The model under review builds one solid part; all positions refer to its coordinate system, in mm. Coordinates: 2 decimals unless noted, no trailing zeros. Loops run counter-clockwise (first coordinate to the right, second up) from the corner with the lowest first, then second, coordinate; pieces in that order, holes last. Notation, with made-up numbers: (-21, -21.75) - (-15, -21.75) arc R13 cw to (-15, -5.75) - close; hole circle Ø9 at (35.5, 67.5). An arc over 180 degrees is marked (long way). Use a Markdown table: item, result. Add a question column.
1) Add section A-A, the plane y = 0. Give the boundary of the cut face in (x, z) (3 decimals), and give its area (3 significant figures).
2) Add section B-B, the plane x = 225. Give the boundary of the cut face in (y, z) (3 decimals).
3) To check wall thickness, follow L1, parallel to Y at x = -225, z = 2; L2, parallel to X at y = 4, z = 3.75; L3, parallel to Y at x = 236, z = 0. State the ranges of each line that lie inside material, in increasing order. Write a range as [from, to].
4) Add section C-C, the plane z = 3. Give the boundary of the cut face in (x, y), and give its area (3 significant figures).
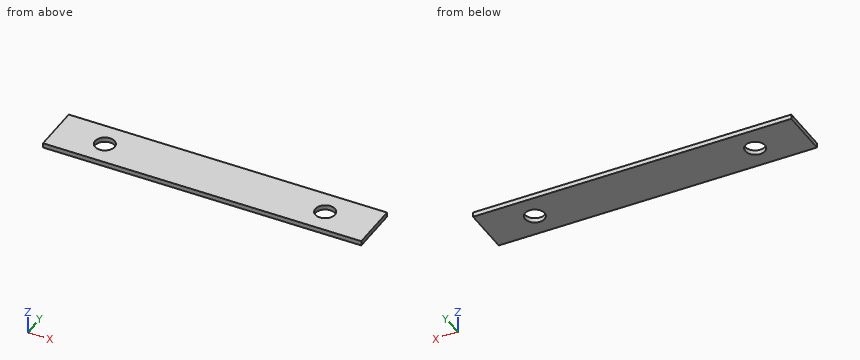
```python
from build123d import *

# Parameters (mm, degrees)
CROQUIS1_W              = 650
CROQUIS1_H              = 100
SALIENTE_EXTRUIR1_DEPTH = 4.765
CROQUIS4_R              = 20
CORTAR_EXTRUIR3_DEPTH   = 15
CROQUIS3_R              = 20
CORTAR_EXTRUIR4_DEPTH   = 15


with BuildPart() as part:
    # Croquis1 → Saliente-Extruir1 (new, symmetric)
    with BuildSketch(Plane.XY):
        Rectangle(CROQUIS1_W, CROQUIS1_H)
    extrude(amount=SALIENTE_EXTRUIR1_DEPTH, both=True)

    # Croquis4 → Cortar-Extruir3 (cut)
    with BuildSketch(Plane(origin=(0, 0, -4.765), x_dir=(-1, 0, 0), z_dir=(0, 0, -1))):
        with Locations((225, 0)):
            Circle(CROQUIS4_R)
    extrude(amount=-CORTAR_EXTRUIR3_DEPTH, mode=Mode.SUBTRACT)

    # Croquis3 → Cortar-Extruir4 (cut)
    with BuildSketch(Plane.XY.offset(4.765)):
        with Locations((225, 0)):
            Circle(CROQUIS3_R)
    extrude(amount=-CORTAR_EXTRUIR4_DEPTH, mode=Mode.SUBTRACT)


solid = part.part
```
From the geometry:
| question | item | result |
|---|---|---|
| 1 | outline | (-325, -4.765) - (-245, -4.765) - (-245, 4.765) - (-325, 4.765) - close; (-205, -4.765) - (205, -4.765) - (205, 4.765) - (-205, 4.765) - close; (245, -4.765) - (325, -4.765) - (325, 4.765) - (245, 4.765) - close |
| 1 | area | 5,430 mm^2 |
| 2 | outline | (-50, -4.765) - (-20, -4.765) - (-20, 4.765) - (-50, 4.765) - close; (20, -4.765) - (50, -4.765) - (50, 4.765) - (20, 4.765) - close |
| 3 | L1 | y = [-50, -20], [20, 50] |
| 3 | L2 | x = [-325, -244.6], [-205.4, 205.4], [244.6, 325] |
| 3 | L3 | y = [-50, -16.7], [16.7, 50] |
| 4 | outline | (-325, -50) - (325, -50) - (325, 50) - (-325, 50) - close; hole circle Ø40 at (-225, 0); hole circle Ø40 at (225, 0) |
| 4 | area | 62,500 mm^2 |
